from build123d import *

# Parameters (mm, degrees)
F0_W      = 180
F0_H      = 95
F1_DEPTH  = 50
F2_W      = 160
F2_H      = 75
F3_DEPTH  = 50.001
F4_W      = 170
F4_H      = 85
F5_DEPTH  = 10
F6_W      = 170
F6_H      = 85
F7_DEPTH  = 10
F8_R      = 3
F9_R      = 5
F10_DEPTH = 10


with BuildPart() as f1:
    # F0 (on Top) → F1 (new body)
    with BuildSketch(Plane.XY):
        with Locations((-2.011862, -11.363395)):
            Rectangle(F0_W, F0_H)
    extrude(amount=F1_DEPTH)

    # F2 (on face) → F3 (cut, through all)
    with BuildSketch(Plane.XY.offset(50)):
        with Locations((-2.011862, -11.363395)):
            Rectangle(F2_W, F2_H)
    extrude(amount=-F3_DEPTH, mode=Mode.SUBTRACT)

    # F4 (on face) → F5 (cut)
    with BuildSketch(Plane.XY.offset(50)):
        with Locations((-2.011862, -11.363395)):
            Rectangle(F4_W, F4_H)
    extrude(amount=-F5_DEPTH, mode=Mode.SUBTRACT)

    # F6 (on face) → F7 (cut)
    with BuildSketch(Plane(origin=(0, 0, 0), x_dir=(1, 0, 0), z_dir=(0, 0, -1))):
        with Locations((-2.011862, 11.363395)):
            Rectangle(F6_W, F6_H)
    extrude(amount=-F7_DEPTH, mode=Mode.SUBTRACT)

    # F8
    f8_edges = [f1.edges().sort_by_distance(p)[0] for p in [
        (-92.011862, -58.863395, 25),
        (87.988138, -58.863395, 25),
        (87.988138, -11.363395, 50),
        (-2.011862, -58.863395, 50),
        (-92.011862, -11.363395, 50),
        (-2.011862, 36.136605, 50),
        (-92.011862, 36.136605, 25),
        (87.988138, 36.136605, 25),
    ]]
    fillet(f8_edges, radius=F8_R)

    # F9 (on face) → F10 (cut, through all)
    with BuildSketch(Plane(origin=(0, 36.136605, 0), x_dir=(-1, 0, 0), z_dir=(0, 1, 0))):
        with Locations((-57.988138, 23.5)):
            Circle(F9_R)
    extrude(amount=-F10_DEPTH, mode=Mode.SUBTRACT)


solid = f1.part
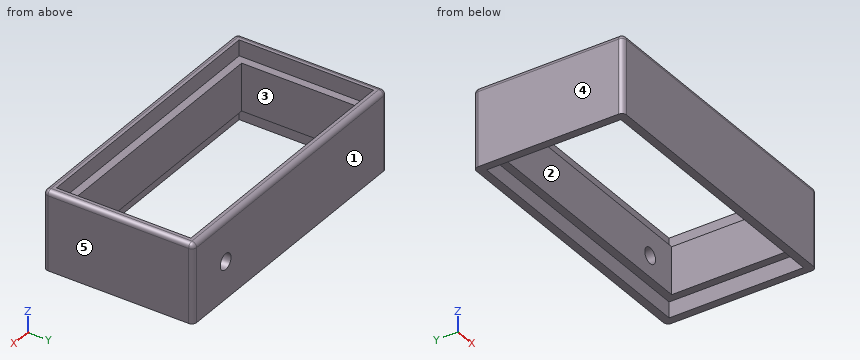
Verification items for the finished model (mm, model axes). Face numbers are marked on the shaded views. A direction names the side the tool comes from. Coordinates: 2 decimals unless noted, no trailing zeros. Write each loop counter-clockwise with the first axis right and the second up, starting at its lowest first coordinate (ties: lowest second). Pieces come first, ordered by that corner, then holes. Notation, with made-up numbers: M 61,50 L 106,50 A26 cw 106,65 Z; hole C 63.25,87 d9. An arc over 180 degrees is marked long. Use a Markdown table: item, result.
Q1. Sectioned sample at D-D, the plane z = 26.5. Record the boundary of the cut face in (x, y).
Reply:
| item | result |
|---|---|
| outline | M -92.01,-55.86 A3 ccw -89.01,-58.86 L 84.99,-58.86 A3 ccw 87.99,-55.86 L 87.99,33.14 A3 ccw 84.99,36.14 L 61.99,36.14 L 61.99,26.14 L 77.99,26.14 L 77.99,-48.86 L -82.01,-48.86 L -82.01,26.14 L 53.99,26.14 L 53.99,36.14 L -89.01,36.14 A3 ccw -92.01,33.14 Z |
Q2. Sectioned sample at B-B, the plane z = 16.5. Record the boundary of the cut face in (x, y).
Reply:
| item | result |
|---|---|
| outline | M -92.01,-55.86 A3 ccw -89.01,-58.86 L 84.99,-58.86 A3 ccw 87.99,-55.86 L 87.99,33.14 A3 ccw 84.99,36.14 L -89.01,36.14 A3 ccw -92.01,33.14 Z; hole M -82.01,-48.86 L 77.99,-48.86 L 77.99,26.14 L -82.01,26.14 Z |
Q3. Sectioned sample at A-A, the plane y = -37. Record the boundary of the cut face in (x, z), plus the area to 3 significant figures.
Reply:
| item | result |
|---|---|
| outline | M -92.01,0 L -87.01,0 L -87.01,10 L -82.01,10 L -82.01,40 L -87.01,40 L -87.01,50 L -89.01,50 A3 ccw -92.01,47 Z; M 77.99,10 L 82.99,10 L 82.99,0 L 87.99,0 L 87.99,47 A3 ccw 84.99,50 L 82.99,50 L 82.99,40 L 77.99,40 Z |
| area | 796 mm² |
Q4. Draft check along X on the marked faces 3, 4 and 5. Enter one of: +X half, -X half, draft (parallel to the pull), parting line (faces both ways), or undercut.
Reply:
| item | result |
|---|---|
| face 3 | undercut |
| face 4 | -X half |
| face 5 | +X half |
Q5. Thickness scan on line 1 (X direction, y = 17, z = 39); line 2 (X direction, y = -14, z = 6); line 3 (Y direction, x = -57, z = 42). Record the ranges inside material, lowest first.
Reply:
| item | result |
|---|---|
| line 1 | x = -92.01 to -82.01, 77.99 to 87.99 |
| line 2 | x = -92.01 to -87.01, 82.99 to 87.99 |
| line 3 | y = -58.86 to -53.86, 31.14 to 36.14 |
Q6. Set-up check for the marked faces 1 and 2: record each of +Z, -Z, +X, -X, +Y, -Y from which the full face is reachable in a straight line by a thin tool's end or side.
Reply:
| item | result |
|---|---|
| face 1 | +Z, -Z, +X, -X, +Y |
| face 2 | +Z, -Z |
Q7. Sectioned sample at C-C, the plane x = 72.5. Record the boundary of the cut face in (y, z).
Reply:
| item | result |
|---|---|
| outline | M -58.86,0 L -53.86,0 L -53.86,10 L -48.86,10 L -48.86,40 L -53.86,40 L -53.86,50 L -55.86,50 A3 ccw -58.86,47 Z; M 26.14,10 L 31.14,10 L 31.14,0 L 36.14,0 L 36.14,47 A3 ccw 33.14,50 L 31.14,50 L 31.14,40 L 26.14,40 Z |
